Check sheet for the modelled part. Datum: model origin and axes. Units: mm. Face numbers are marked on the shaded views. Coordinates: 2 decimals unless noted, no trailing zeros. Loops run counter-clockwise (first coordinate to the right, second up) from the corner with the lowest first, then second, coordinate; pieces in that order, holes last. Notation, with made-up numbers: (11, -37.5) -> (24, -37.5) arc R26 cw to (24, -18.5) -> close; hole circle Ø8 at (-16.5, 2). An arc over 180 degrees is marked (long way). Use CSV: the item, a comma, the result in double quotes. Start each with the question number.
1. Sectioned sample at A-A, the plane x = -218. Record the cut outline in (y, z), and give its area (3 significant figures).
2. Gauge pin test, flat ends, axial feed: pin 1 (12 mm diameter, centred on x = -80, z = 824, fed in from -Y); pin 2 (10 mm diameter, centred on x = -237.5, z = 979, fed in from +Y); pin 3 (8 mm diameter, centred on x = -73.5, z = 1731.5, fed in from -Y). Record the tip position at first contact, or that the pin passes through.
3. Thickness scan on L1, parallel to X at y = 168, z = 123; L2, parallel to Y at x = -383, z = 1377; L3, parallel to Y at x = 282.5, z = 709. Record the ranges inside material, lowest first.
4. Sectioned sample at B-B, the plane z = 1677.5. Record the cut outline in (x, y), and give its area (3 significant figures).
5. Release check for a two-part mould opening along X. For the marked faces 1, 2 and 3 record: pulls with the +X half, pulls with the -X half, needs draft (parallel to the pull), parting line crosses it, or undercut.
```python
from build123d import *

# Parameters (mm, degrees)
F2_DEPTH = 609.6
F3_START = 542.29
F3_DEPTH = 6.35


# Not quite as in the source:
# - a length typed as a fraction of an inch, garbled in the dataset ("3 / 203.2 mm" for 3/8 in), is restored


with BuildPart() as f2:
    # F0 (on Right) → F2 (new body, symmetric)
    with BuildSketch(Plane.YZ):
        Polygon((-6.5879129879, 0.4606717526), (0, 0), (170.0941855777, 2432.4601801536), (163.4740592827, 2432.4601801536), align=None)
    extrude(amount=F2_DEPTH, both=True)

    # F1 (on Right) → F3 (join)
    with BuildSketch(Plane.YZ.offset(F3_START)):
        with BuildLine():
            Line((-43.1832319469, -7.9277986727), (-50.8, -101.6))
            Line((-50.8, -101.6), (406.4, -101.6))
            add(Edge.make_bspline(
                [(128.1419030371, 1060.091129987), (120.5565482378, 184.9341541529), (188.3697360754, 77.5789916515), (406.4, -101.6)],
                knots=[0, 0, 0, 0, 1194.5517360148, 1194.5517360148, 1194.5517360148, 1194.5517360148], degree=3))
            Line((128.1419030371, 1060.091129987), (78.1502050281, 1117.6))
            Line((78.1502050281, 1117.6), (0, 0))
            Line((0, 0), (-6.5879129879, 0.4606717526))
            Line((-6.5879129879, 0.4606717526), (-4.8439852716, 25.4))
            Line((-4.8439852716, 25.4), (-43.1832319469, -7.9277986727))
        make_face()
    extrude(amount=F3_DEPTH)

    # F4: F2 across plane


with BuildPart() as f2_1:
    add(f2.part)
    add(f2.part.mirror(Plane.YZ))


solid = f2_1.part
```
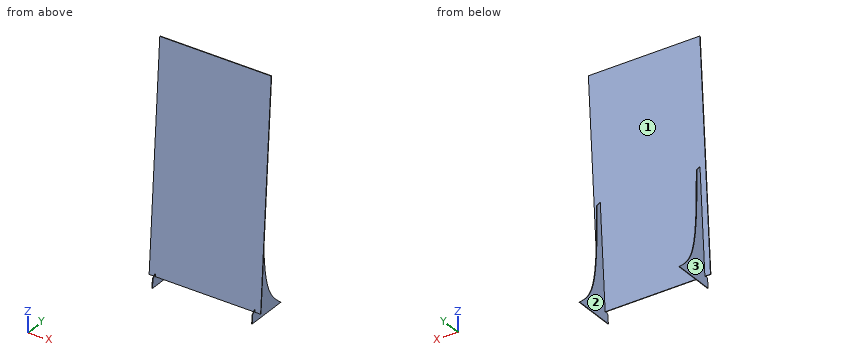
Completed:
1,outline,"(-6.59, 0.46) -> (0, 0) -> (170.09, 2432.46) -> (163.47, 2432.46) -> close"
1,area,"16,100 mm²"
2,pin 1,"y = 50.58"
2,pin 2,"y = 68.81"
2,pin 3,"y = 114.18"
3,L1,"-548.64 to -542.29, 542.29 to 548.64"
3,L2,"89.67 to 96.29"
3,L3,"42.96 to 49.58"
4,outline,"(-609.6, 110.68) -> (609.6, 110.68) -> (609.6, 117.3) -> (-609.6, 117.3) -> close"
4,area,"8,070 mm²"
5,face 1,"undercut"
5,face 2,"undercut"
5,face 3,"pulls with the -X half"
